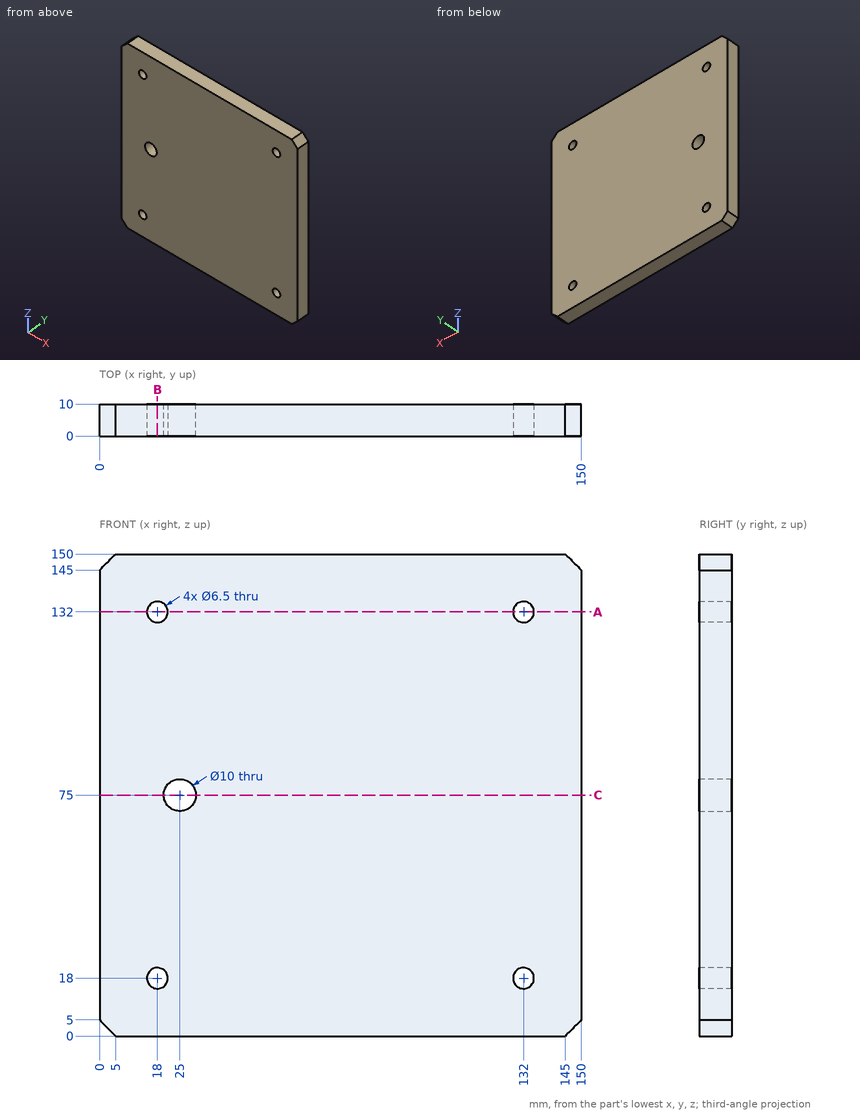
Job drawing, mm, ordinate dimensions from the low corner. One solid piece. Round coordinates to 2 decimals unless told otherwise and drop trailing zeros. Loops run counter-clockwise (first coordinate to the right, second up) from the corner with the lowest first, then second, coordinate; pieces in that order, holes last. Notation, with made-up numbers: M 75.25,56.5 L 96.25,56.5 A14 cw 96.25,63.5 Z; hole C 63.25,41.5 d4. An arc over 180 degrees is marked long. One line per question, with ' | ' between items. Start each with the question number.
Item 1: Cut at A-A, the plane z = 132. Write the cut outline in (x, y).
Item 2: Cut at B-B, the plane x = 18. Write the cut outline in (y, z).
Item 3: Wall check: line 1 (X direction, y = 2, z = 132); line 2 (Z direction, x = 16, y = 9). Give the ranges that are in metal, low to high.
Item 4: Cut at C-C, the plane z = 75. Write the cut outline in (x, y).
Responses:
1) outline: M 0,0 L 14.75,0 L 14.75,10 L 0,10 Z; M 21.25,0 L 128.75,0 L 128.75,10 L 21.25,10 Z; M 135.25,0 L 150,0 L 150,10 L 135.25,10 Z
2) outline: M 0,0 L 10,0 L 10,14.75 L 0,14.75 Z; M 0,21.25 L 10,21.25 L 10,128.75 L 0,128.75 Z; M 0,135.25 L 10,135.25 L 10,150 L 0,150 Z
3) line 1: x = 0 to 14.75, 21.25 to 128.75, 135.25 to 150 | line 2: z = 0 to 15.44, 20.56 to 129.44, 134.56 to 150
4) outline: M 0,0 L 20,0 L 20,10 L 0,10 Z; M 30,0 L 150,0 L 150,10 L 30,10 Z
